Could you check a few things on this drawing? It's one solid part, dimensions in mm from its lowest x, y, z. Round coordinates to 2 decimals unless told otherwise and drop trailing zeros. Write each loop counter-clockwise with the first axis right and the second up, starting at its lowest first coordinate (ties: lowest second). Pieces come first, ordered by that corner, then holes. Notation, with made-up numbers: (36.25, 13) -> (68.25, 13) arc R32 cw to (68.25, 41) -> close; hole circle Ø1 at (-5, 2.5). An arc over 180 degrees is marked (long way). Answer in a Markdown table with one row per item.
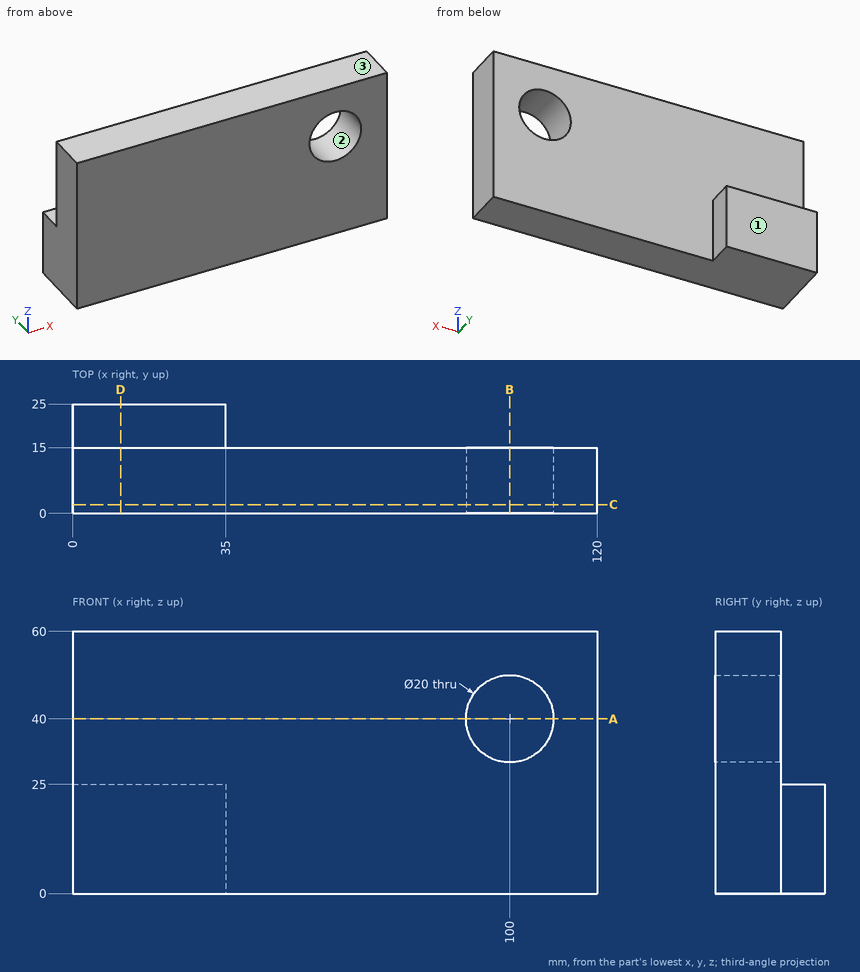
1) We'd pull the mould along Z, two halves only. Please class the marked faces 1, 2 and 3: +Z half, -Z half, draft (parallel to the pull), parting line (faces both ways), or undercut.
Response:
| item | result |
|---|---|
| face 1 | draft |
| face 2 | undercut |
| face 3 | +Z half |
2) I want a section at A-A, the plane z = 40. List the corners of the cut face in (x, y) for me.
Response:
| item | result |
|---|---|
| outline | (0, 0) -> (90, 0) -> (90, 15) -> (0, 15) -> close; (110, 0) -> (120, 0) -> (120, 15) -> (110, 15) -> close |
3) For pin 1 (10 mm diameter, centred on x = 77.5, z = 40.5, fed in from +Y); pin 2 (5 mm diameter, centred on x = 16, y = 20.5, fed in from +Z); pin 3 (4 mm diameter, centred on y = 21.5, z = 12, fed in from +X), each with a flat end and sliding along its axis, tell me the tip position at first contact or that it passes through.
Response:
| item | result |
|---|---|
| pin 1 | stops at y = 15 |
| pin 2 | stops at z = 25 |
| pin 3 | stops at x = 35 |
4) I want a section at D-D, the plane x = 11. List the corners of the cut face in (y, z) for me.
Response:
| item | result |
|---|---|
| outline | (0, 0) -> (25, 0) -> (25, 25) -> (15, 25) -> (15, 60) -> (0, 60) -> close |
5) I want a section at C-C, the plane y = 2. List the corners of the cut face in (x, z) for me, and give its area (3 significant figures).
Response:
| item | result |
|---|---|
| outline | (0, 0) -> (120, 0) -> (120, 60) -> (0, 60) -> close; hole circle Ø20 at (100, 40) |
| area | 6,890 mm^2 |
6) I want a section at B-B, the plane x = 100. List the corners of the cut face in (y, z) for me, and give its area (3 significant figures).
Response:
| item | result |
|---|---|
| outline | (0, 0) -> (15, 0) -> (15, 30) -> (0, 30) -> close; (0, 50) -> (15, 50) -> (15, 60) -> (0, 60) -> close |
| area | 600 mm^2 |
7) I need wall thicknesses on line 1 (X direction, y = 11.25, z = 40); line 2 (Y direction, x = 19, z = 52); line 3 (Z direction, x = 96, y = 6.75). Which ranges of each line are inside material? Lowest first, please. Write a range as [from, to].
Response:
| item | result |
|---|---|
| line 1 | x = [0, 90], [110, 120] |
| line 2 | y = [0, 15] |
| line 3 | z = [0, 30.83], [49.17, 60] |
